from build123d import *

# Parameters (mm, degrees)
SKETCH_W        = 224
SKETCH_H        = 344
PAD_DEPTH       = 18
SKETCH001_R     = 6
POCKET_DEPTH    = 7
SKETCH002_R     = 3.1
POCKET001_DEPTH = 11
FILLET_R        = 6
FILLET001_R     = 6
FILLET002_R     = 6
FILLET003_R     = 6
FILLET004_R     = 12


with BuildPart() as part:
    # Sketch → Pad (new body)
    with BuildSketch(Plane.XY):
        with Locations((112, 172)):
            Rectangle(SKETCH_W, SKETCH_H)
    extrude(amount=PAD_DEPTH)

    # Sketch001 (on Face6 of Pad) → Pocket (cut)
    with BuildSketch(Plane.XY.offset(18)):
        with Locations((112, 322)):
            Circle(SKETCH001_R)
        with Locations((22, 270)):
            Circle(SKETCH001_R)
        with Locations((22, 74)):
            Circle(SKETCH001_R)
        with Locations((202, 234)):
            Circle(SKETCH001_R)
        with Locations((202, 110)):
            Circle(SKETCH001_R)
        with Locations((112, 22)):
            Circle(SKETCH001_R)
        with Locations((22, 234)):
            Circle(SKETCH001_R)
        with Locations((22, 110)):
            Circle(SKETCH001_R)
        with Locations((202, 270)):
            Circle(SKETCH001_R)
        with Locations((202, 74)):
            Circle(SKETCH001_R)
    extrude(amount=-POCKET_DEPTH, mode=Mode.SUBTRACT)

    # Sketch002 (on Face4 of Pocket) → Pocket001 (cut)
    with BuildSketch(Plane(origin=(0, 0, 0), x_dir=(1, 0, 0), z_dir=(0, 0, -1))):
        with Locations((112, -22)):
            Circle(SKETCH002_R)
        with Locations((22, -74)):
            Circle(SKETCH002_R)
        with Locations((22, -110)):
            Circle(SKETCH002_R)
        with Locations((22, -234)):
            Circle(SKETCH002_R)
        with Locations((22, -270)):
            Circle(SKETCH002_R)
        with Locations((202, -74)):
            Circle(SKETCH002_R)
        with Locations((202, -110)):
            Circle(SKETCH002_R)
        with Locations((202, -234)):
            Circle(SKETCH002_R)
        with Locations((202, -270)):
            Circle(SKETCH002_R)
        with Locations((112, -322)):
            Circle(SKETCH002_R)
    extrude(amount=-POCKET001_DEPTH, mode=Mode.SUBTRACT)

    # Fillet
    fillet_edges = [part.edges().sort_by_distance(p)[0] for p in [
        (224, 0, 9),
    ]]
    fillet(fillet_edges, radius=FILLET_R)

    # Fillet001
    fillet001_edges = [part.edges().sort_by_distance(p)[0] for p in [
        (0, 0, 9),
    ]]
    fillet(fillet001_edges, radius=FILLET001_R)

    # Fillet002
    fillet002_edges = [part.edges().sort_by_distance(p)[0] for p in [
        (0, 344, 9),
    ]]
    fillet(fillet002_edges, radius=FILLET002_R)

    # Fillet003
    fillet003_edges = [part.edges().sort_by_distance(p)[0] for p in [
        (224, 344, 9),
    ]]
    fillet(fillet003_edges, radius=FILLET003_R)

    # Fillet004
    fillet004_edges = [part.edges().sort_by_distance(p)[0] for p in [
        (112, 0, 18),
        (222.242641, 1.757359, 18),
        (1.757359, 1.757359, 18),
        (0, 172, 18),
        (1.757359, 342.242641, 18),
        (112, 344, 18),
        (222.242641, 342.242641, 18),
        (224, 172, 18),
    ]]
    fillet(fillet004_edges, radius=FILLET004_R)


solid = part.part
Model file for the job. Use its own axes, mm. A direction names the side the tool comes from. Give positions to 0.01 mm unless a question says otherwise; leave off trailing zeros. Order: outer loops, then holes, each group sorted by start corner. A loop starts at its lowest first (then second) coordinate and runs counter-clockwise, first axis right, second up. Notation, with made-up numbers: M 73,56.25 L 115,56.25 A6 ccw 115,67.25 Z; hole C 2.25,1.5 d3. An arc over 180 degrees is marked long. Put each result on its own line as item: value. Start each with the question number.
(1) Band-saw the part on B-B on z = 14.25. Count the separate pieces of the cut face and the enclosed holes in it, then the cut area to 3 significant figures.
(2) Drill centre lines: L1, parallel to Y at x = 112, z = 3.25; L2, parallel to X at y = 270, z = 13; L3, parallel to Y at x = 202, z = 13. Where is each one in solid material? Low to high. Write a range as [from, to].
(3) Pull direction X, two halves, no side cores. Call faces 1 (the face through (115, 319, 11)), 2 (the face through (25, 107, 11)), 3 (the face through (110, 174, 0)): released by +X, released by -X, zero draft, split by the parting line, or undercut.
(4) Pin check, flat tips, straight feed: pin 1 Ø8 at (y, z) = (262.5, 12) entering from -X; pin 2 Ø3 at (y, z) = (303, 8) entering from +X; pin 3 Ø3.5 at (x, y) = (204, 271.5) entering from +Z. Stop position of each tip, or through.
(5) Band-saw the part on A-A on y = 85.5. Give the cut face in (x, z).
(6) Tool access for faces 4 (the face through (205, 107, 11)), 5 (the face through (19.72, 71.9, 5.42)): list every direction of +Z, -Z, +X, -X, +Y, -Y with a clear straight run to the whole face (end or side of a thin tool).
Results below:
1. separate pieces: 1
1. enclosed holes: 10
1. area: 72,200 mm2
2. L1: y = [0, 18.9], [25.1, 318.9], [325.1, 344]
2. L2: x = [2.25, 16], [28, 196], [208, 221.75]
2. L3: y = [2.25, 68], [80, 104], [116, 228], [240, 264], [276, 341.75]
3. face 1: undercut
3. face 2: undercut
3. face 3: zero draft
4. pin 1: stops at x = 0.17
4. pin 2: stops at x = 223.99
4. pin 3: stops at z = 11
5. outline: M 0,0 L 224,0 L 224,6 A12 ccw 212,18 L 12,18 A12 ccw 0,6 Z
6. face 4: +Z
6. face 5: +Z, -Z
